from build123d import *

# Parameters (mm, degrees)
SKETCH2_R          = 4.5
CUT_EXTRUDE1_DEPTH = 127.479115352
CIRPATTERN1_COUNT  = 8
SKETCH3_R          = 5
CUT_EXTRUDE2_DEPTH = 70


with BuildPart() as part:
    # Sketch1 → Revolve1 (revolve)
    with BuildSketch(Plane(origin=(0, 0, 0), x_dir=(0, 0, -1), z_dir=(1, 0, 0)), mode=Mode.PRIVATE) as revolve1_sk:
        Polygon((-9.502538071, 5.664974619), (-81.502538071, 5.664974619), (-81.502538071, 13.414974619), (-79.502538071, 13.414974619), (-79.502538071, 33.414974619), (-71.002538071, 33.414974619), (-71.002538071, 15.914974619), (-9.502538071, 15.914974619), align=None)
    revolve(revolve1_sk.sketch.rotate(Axis((0, -26.585025381, 81.502538071), (0, 0, -1)), 90), axis=Axis((0, -26.585025381, 81.502538071), (0, 0, -1)))

    # Sketch2 → Cut-Extrude1 (cut, symmetric)
    with BuildSketch(Plane.XY.offset(79.502538071)):
        with Locations((51, -26.585025381)):
            Circle(SKETCH2_R)
    cut_extrude1 = extrude(amount=CUT_EXTRUDE1_DEPTH, both=True, mode=Mode.SUBTRACT)

    # CirPattern1: Cut-Extrude1 ×8 about axis
    cirpattern1_axis = Axis((0, -26.585025381, 0), (0, 0, 1))
    for i in range(1, CIRPATTERN1_COUNT):
        add(cut_extrude1.rotate(cirpattern1_axis, i * 360 / CIRPATTERN1_COUNT), mode=Mode.SUBTRACT)

    # Sketch3 → Cut-Extrude2 (cut)
    with BuildSketch(Plane(origin=(0, 0, 0), x_dir=(0, 0, -1), z_dir=(1, 0, 0))):
        with Locations(Location((-39.502538071, -26.585025381, 0), (0, 0, 180))):
            Circle(SKETCH3_R)
    extrude(amount=CUT_EXTRUDE2_DEPTH, mode=Mode.SUBTRACT)


solid = part.part
Part model, mm, in its own coordinate system. A direction names the side the tool comes from. Coordinates: 2 decimals unless noted, no trailing zeros. Order: outer loops, then holes, each group sorted by start corner. A loop starts at its lowest first (then second) coordinate and runs counter-clockwise, first axis right, second up.
(1) Slice it at B-B, the plane y = -13.5. Write the cut outline in (x, z), and give its area (3 significant figures).
Check sheet entries:
outline: (-58.56, 71) - (-40.44, 71) - (-40.44, 9.5) - (-29.48, 9.5) - (-29.48, 81.5) - (-37.8, 81.5) - (-37.8, 79.5) - (-58.56, 79.5) - close; (29.48, 9.5) - (40.44, 9.5) - (40.44, 71) - (58.56, 71) - (58.56, 79.5) - (37.8, 79.5) - (37.8, 81.5) - (29.48, 81.5) - close
area: 1,880 mm2
(2) Pull direction Y, two halves, no side cores. Call faces 6 (the face through (35.87, -58.15, 75.31)), 7 (the face through (-39.96, -28.34, 80.49)), 8 (the face through (27, -45, 81.503)): pulls with the +Y half, pulls with the -Y half, needs draft (parallel to the pull), parting line crosses it, or undercut.
Check sheet entries:
face 6: undercut
face 7: parting line crosses it
face 8: needs draft
(3) Slice it at C-C, the plane x = 51. Write the cut outline in (y, z).
Check sheet entries:
outline: (-58.19, 71) - (-31.09, 71) - (-31.09, 79.5) - (-58.19, 79.5) - close; (-22.09, 71) - (5.02, 71) - (5.02, 79.5) - (-22.09, 79.5) - close
(4) Tool access for faces 1 (the face through (-9.213, 14.904, 39.822)), 2 (the face through (37.106, -31.542, 38.852)), 3 (the face through (38.48, 5.68, 75.31)), 4 (the face through (1, -67, 79.503)), 5 (the face through (16, -55, 9.503)): list every direction of +Z, -Z, +X, -X, +Y, -Y with a clear straight run to the whole face (end or side of a thin tool).
Check sheet entries:
face 1: -Z
face 2: +X
face 3: +Z, -Z
face 4: +Z
face 5: -Z, +X, -X, +Y, -Y
(5) Slice it at D-D, the plane y = -56.5. Write the cut outline in (x, z), and give its area (3 significant figures).
Check sheet entries:
outline: (-52.01, 71) - (-30.19, 71) - (-30.19, 9.5) - (-12.05, 9.5) - (-12.05, 81.5) - (-26.55, 81.5) - (-26.55, 79.5) - (-52.01, 79.5) - close; (12.05, 9.5) - (30.19, 9.5) - (30.19, 71) - (52.01, 71) - (52.01, 79.5) - (26.55, 79.5) - (26.55, 81.5) - (12.05, 81.5) - close
area: 2,970 mm2
(6) Pin check, flat tips, straight feed: pin 1 Ø7 at (x, y) = (-51, -26.59) entering from -Z; pin 2 Ø9 at (y, z) = (-26.59, 39.5) entering from -X; pin 3 Ø8 at (x, z) = (-28.5, 46.5) entering from +Y; pin 4 Ø3 at (x, z) = (-3.5, 57) entering from -Y. Stop position of each tip, or through.
Check sheet entries:
pin 1: passes through
pin 2: stops at x = -42.5
pin 3: stops at y = 8.14
pin 4: stops at y = -69.04
(7) Slice it at A-A, the plane x = 0. Write the cut outline in (y, z).
Check sheet entries:
outline: (-86.59, 71) - (-82.09, 71) - (-82.09, 79.5) - (-86.59, 79.5) - close; (-73.09, 71) - (-69.09, 71) - (-69.09, 9.5) - (-58.84, 9.5) - (-58.84, 81.5) - (-66.59, 81.5) - (-66.59, 79.5) - (-73.09, 79.5) - close; (5.66, 9.5) - (15.91, 9.5) - (15.91, 71) - (19.91, 71) - (19.91, 79.5) - (13.41, 79.5) - (13.41, 81.5) - (5.66, 81.5) - close; (28.91, 71) - (33.41, 71) - (33.41, 79.5) - (28.91, 79.5) - close
(8) Probe L1, parallel to X at y = 2, z = 54; L2, parallel to X at y = -8, z = 76.5; L3, parallel to Y at x = 12.5, z = 35. List the from-to ranges inside material, lowest first.
Check sheet entries:
L1: x = -31.45 to -14.93, 14.93 to 31.45
L2: x = -57.05 to -26.36, 26.36 to 57.05
L3: y = -67.21 to -56.31, 3.14 to 14.04
